```python
from build123d import *

# Parameters (mm, degrees)
BOSS_EXTRUDE1_START        = -0.486816485
BOSS_EXTRUDE1_DEPTH        = 3.661816485
SKETCH2_W                  = 23.8125
SKETCH2_H                  = 3.175
BOSS_EXTRUDE2_DEPTH        = 25.4
CUT_EXTRUDE1_DEPTH         = 79.943753108
CUT_EXTRUDE1_DEPTH_BACK    = 79.943753108
SKETCH3_R                  = 3.175
CUT_EXTRUDE2_DEPTH         = 76.643257039
CUT_EXTRUDE2_DEPTH_BACK    = 76.643257039
SKETCH6_R                  = 3.175
CUT_EXTRUDE3_DEPTH         = 79.943753108
CUT_EXTRUDE3_DEPTH_BACK    = 79.943753108
SKETCH7_W                  = 26.9875
SKETCH7_H                  = 3.175
FILLET1_R                  = 3.175
CONVERT_SOLID1_DEPTH       = 50.8
CONVERT_SOLID1_START       = 25.4
CONVERT_SOLID1_2_OUTLINE_W = 7.9375
CONVERT_SOLID1_2_OUTLINE_H = 3.175
CONVERT_SOLID1_2_DEPTH     = 1.5875
CONVERT_SOLID1_START_2     = 26.9875
CONVERT_SOLID1_3_DEPTH     = 23.8125
CONVERT_SOLID1_4_DEPTH     = 23.8125


# Read off the part's stored shape, not the designer's step: Convert-Solid1
with BuildPart() as part:
    # Sketch1 → Boss-Extrude1 (new body)
    with BuildSketch(Plane.XY.offset(BOSS_EXTRUDE1_START)):
        Polygon((50.8, 6.35), (25.4, 50.8), (0, 50.8), (0, 0), (50.8, 0), align=None)
    boss_extrude1 = extrude(amount=BOSS_EXTRUDE1_DEPTH)

    # Sketch2 → Boss-Extrude2 (add)
    with BuildSketch(Plane(origin=(0, 0, -0.486816485), x_dir=(-1, 0, 0), z_dir=(0, 0, -1))):
        with Locations((-38.89375, 1.5875)):
            Rectangle(SKETCH2_W, SKETCH2_H)
    extrude(amount=BOSS_EXTRUDE2_DEPTH)

    # Mirror1: Boss-Extrude1 across plane
    add(boss_extrude1.mirror(Plane(origin=(0, 0, -13.186816485), x_dir=(1, 0, 0), z_dir=(0, 0, -1))))

    # Sketch3 → Cut-Extrude1 (cut, two sides: drawn at the far end of the back side and taken through both)
    with BuildSketch(Plane.XY.offset(3.175).offset(-CUT_EXTRUDE1_DEPTH_BACK)):
        with Locations((12.7, 12.7)):
            Circle(SKETCH3_R)
        with Locations((12.7, 25.4)):
            Circle(SKETCH3_R)
        with Locations((12.7, 38.1)):
            Circle(SKETCH3_R)
    extrude(amount=CUT_EXTRUDE1_DEPTH + CUT_EXTRUDE1_DEPTH_BACK, mode=Mode.SUBTRACT)

    # Sketch6 → Cut-Extrude2 (cut, two sides: drawn at the far end of the back side and taken through both)
    with BuildSketch(Plane(origin=(0, 3.175, 0), x_dir=(1, 0, 0), z_dir=(0, 1, 0)).offset(-CUT_EXTRUDE2_DEPTH_BACK)):
        with Locations(Location((38.1, 13.186816485, 0), (0, 0, 270))):
            Circle(SKETCH6_R)
    extrude(amount=CUT_EXTRUDE2_DEPTH + CUT_EXTRUDE2_DEPTH_BACK, mode=Mode.SUBTRACT)

    # Sketch7 → Cut-Extrude3 (cut, two sides: drawn at the far end of the back side and taken through both)
    with BuildSketch(Plane(origin=(0, 0, -29.54863297), x_dir=(-1, 0, 0), z_dir=(0, 0, -1)).offset(-CUT_EXTRUDE3_DEPTH_BACK)):
        with Locations((-13.49375, 1.5875)):
            Rectangle(SKETCH7_W, SKETCH7_H)
    extrude(amount=CUT_EXTRUDE3_DEPTH + CUT_EXTRUDE3_DEPTH_BACK, mode=Mode.SUBTRACT)

    # Fillet1
    fillet1_edges = [part.edges().sort_by_distance(p)[0] for p in [
        (38.89375, 0, -29.54863297),
        (38.89375, 0, 3.175),
    ]]
    fillet(fillet1_edges, radius=FILLET1_R)

    # Convert-Solid1 outline → Convert-Solid1 (cut)
    with BuildSketch(Plane.YZ):
        with BuildLine():
            Line((50.8, -29.061816485), (3.175, -29.061816485))
            Line((3.175, -29.061816485), (3.175, -28.2110778))
            ThreePointArc((3.175, -28.2110778), (0.850738686, -25.886816486), (0, -22.711816485))
            Line((0, -22.711816485), (0, -26.37363297))
            ThreePointArc((0, -26.37363297), (0.92993597, -28.618697), (3.175, -29.54863297))
            Line((3.175, -29.54863297), (50.8, -29.54863297))
            Line((50.8, -29.54863297), (50.8, -29.061816485))
        make_face()
        with BuildLine():
            Line((0, 0), (0, -3.661816485))
            ThreePointArc((0, -3.661816485), (0.850738686, -0.486816484), (3.175, 1.83744483))
            Line((3.175, 1.83744483), (3.175, 2.688183515))
            Line((3.175, 2.688183515), (50.8, 2.688183515))
            Line((50.8, 2.688183515), (50.8, 3.175))
            Line((50.8, 3.175), (3.175, 3.175))
            ThreePointArc((3.175, 3.175), (0.92993597, 2.24506403), (0, 0))
        make_face()
    extrude(amount=CONVERT_SOLID1_DEPTH, mode=Mode.SUBTRACT)

    # Convert-Solid1 2 outline → Convert-Solid1 2 (cut)
    with BuildSketch(Plane.YZ.offset(CONVERT_SOLID1_START)):
        with Locations((7.14375, -27.474316485)):
            Rectangle(CONVERT_SOLID1_2_OUTLINE_W, CONVERT_SOLID1_2_OUTLINE_H)
        with Locations((7.14375, 1.100683515)):
            Rectangle(CONVERT_SOLID1_2_OUTLINE_W, CONVERT_SOLID1_2_OUTLINE_H)
    extrude(amount=CONVERT_SOLID1_2_DEPTH, mode=Mode.SUBTRACT)

    # Convert-Solid1 3 outline → Convert-Solid1 3 (cut)
    with BuildSketch(Plane.YZ.offset(CONVERT_SOLID1_START_2)):
        with BuildLine():
            Line((3.175, -29.061816485), (6.35, -29.061816485))
            ThreePointArc((6.35, -29.061816485), (4.706499064, -28.845445482), (3.175, -28.2110778))
            Line((3.175, -28.2110778), (3.175, -29.061816485))
        make_face()
        with BuildLine():
            Line((3.175, 2.688183515), (3.175, 1.83744483))
            ThreePointArc((3.175, 1.83744483), (4.706499064, 2.471812512), (6.35, 2.688183515))
            Line((6.35, 2.688183515), (3.175, 2.688183515))
        make_face()
    extrude(amount=CONVERT_SOLID1_3_DEPTH, mode=Mode.SUBTRACT)

    # Convert-Solid1 4 outline → Convert-Solid1 4 (add)
    with BuildSketch(Plane.YZ.offset(CONVERT_SOLID1_START_2)):
        with BuildLine():
            Line((3.175, -25.886816485), (6.35, -25.886816485))
            ThreePointArc((6.35, -25.886816485), (4.10493597, -24.956880515), (3.175, -22.711816485))
            Line((3.175, -22.711816485), (3.175, -25.886816485))
        make_face()
        with BuildLine():
            Line((3.175, -0.486816485), (3.175, -3.661816485))
            ThreePointArc((3.175, -3.661816485), (4.10493597, -1.416752455), (6.35, -0.486816485))
            Line((6.35, -0.486816485), (3.175, -0.486816485))
        make_face()
    extrude(amount=CONVERT_SOLID1_4_DEPTH)


solid = part.part
```
Design review of the part built by this model. Coordinates are the model's own, in mm. A direction names the side the tool comes from. Give positions to 0.01 mm unless a question says otherwise; leave off trailing zeros. Loops run counter-clockwise (first coordinate to the right, second up) from the corner with the lowest first, then second, coordinate; pieces in that order, holes last. Notation, with made-up numbers: (83, 6) -> (100, 6) arc R27 cw to (100, 38) -> close; hole circle Ø7 at (-32, -9.5). An arc over 180 degrees is marked (long way). Write each question's results on one line, items separated by ' | '.
Q1. The part is to be moulded in two halves that separate along Z. For faces 1 (the face through (13, 50.8, -27)), 2 (the face through (19, 27, -29.062)), 3 (the face through (19, 27, -0.487)), say which applies: +Z half, -Z half, draft (parallel to the pull), parting line (faces both ways), or undercut.
Reply:
face 1: draft | face 2: -Z half | face 3: undercut
Q2. Machinability: for faces 4 (the face through (13, 3.175, 1)), 5 (the face through (38.73, 4.13, -24.98)), 6 (the face through (26, 11.112, -27)), 7 (the face through (0, 27, 1)), 8 (the face through (13, 50.8, 1)), which of the approach directions +Z, -Z, +X, -X, +Y, -Y give a long, thin tool a straight path to every point of the face, cutting with its end or side? Answer none if there is none.
Reply:
face 4: +Z, -Z, -X, -Y | face 5: +X, -X, +Y | face 6: +Z, -Z, -Y | face 7: +Z, -Z, -X, +Y, -Y | face 8: +Z, -Z, +X, -X, +Y
Q3. Take a section at A-A, the plane x = 8.5. Write out the cut boundary in (y, z) (3 decimals), plus the area to 3 significant figures.
Reply:
outline: (3.175, -29.062) -> (50.8, -29.062) -> (50.8, -25.887) -> (3.175, -25.887) -> close; (3.175, -0.487) -> (50.8, -0.487) -> (50.8, 2.688) -> (3.175, 2.688) -> close | area: 302 mm²
Q4. Take a section at D-D, the plane x = 47.5. Write out the cut boundary in (y, z) (3 decimals).
Reply:
outline: (0, -22.712) arc R6.35 ccw to (6.35, -29.062) -> (12.125, -29.062) -> (12.125, -25.887) -> (6.35, -25.887) arc R3.175 cw to (3.175, -22.712) -> (3.175, -3.662) arc R3.175 cw to (6.35, -0.487) -> (12.125, -0.487) -> (12.125, 2.688) -> (6.35, 2.688) arc R6.35 ccw to (0, -3.662) -> close
Q5. Take a section at C-C, the plane y = 12.7. Write out the cut boundary in (x, z) (3 decimals), plus the area to 3 significant figures.
Reply:
outline: (0, -29.062) -> (9.525, -29.062) -> (9.525, -25.887) -> (0, -25.887) -> close; (0, -0.487) -> (9.525, -0.487) -> (9.525, 2.688) -> (0, 2.688) -> close; (15.875, -29.062) -> (47.171, -29.062) -> (47.171, -25.887) -> (15.875, -25.887) -> close; (15.875, -0.487) -> (47.171, -0.487) -> (47.171, 2.688) -> (15.875, 2.688) -> close | area: 259 mm²
Q6. For pin 1 Ø0.5 at (x, z) = (26, 0.5) entering from -Y; pin 2 Ø8.5 at (x, z) = (38.1, -13.19) entering from +Y (3 decimals); pin 3 Ø10 at (y, z) = (26, -8) entering from +X; pin 4 Ø12 at (y, z) = (4.5, -16) entering from -X, all flat-tipped, find the tip position at first contact; note any pin that passes through.
Reply:
pin 1: stops at y = 11.11 | pin 2: stops at y = 3.175 | pin 3: passes through | pin 4: stops at x = 26.99
Q7. Wall thickness on L1, parallel to Y at x = 12.7, z = 1.7 (3 decimals); L2, parallel to Z at x = 9.5, y = 4.5; L3, parallel to Y at x = 25, z = 0 (3 decimals): over which ranges is each line inside the solid? List them lowest first.
Reply:
L1: y = 3.175 to 9.525, 15.875 to 22.225, 28.575 to 34.925, 41.275 to 50.8 | L2: z = -29.06 to -25.89, -0.49 to 2.69 | L3: y = 3.175 to 50.8
Q8. Take a section at B-B, the plane y = 44.5. Write out the cut boundary in (x, z), plus the area to 3 significant figures.
Reply:
outline: (0, -29.06) -> (29, -29.06) -> (29, -25.89) -> (0, -25.89) -> close; (0, -0.49) -> (29, -0.49) -> (29, 2.69) -> (0, 2.69) -> close | area: 184 mm²
